Geometry check sheet. Reference: the model listing, model coordinates, mm. Face numbers are marked on the shaded views. A direction names the side the tool comes from. Give positions to 0.01 mm unless a question says otherwise; leave off trailing zeros. Write each loop counter-clockwise with the first axis right and the second up, starting at its lowest first coordinate (ties: lowest second). Pieces come first, ordered by that corner, then holes. Notation, with made-up numbers: (36.25, 36.5) -> (95.25, 36.5) arc R29 ccw to (95.25, 61.5) -> close; hole circle Ø5 at (-35.5, 89). An arc over 180 degrees is marked (long way). One line per item, written item: value.
from build123d import *

# Parameters (mm, degrees)
F0_W      = 200
F0_H      = 56.94
F0_W_2    = 5
F0_H_2    = 4.2824763805
F1_DEPTH  = 0.5
F2_DEPTH  = 0.501
F3_W      = 1
F3_H      = 24.6360383326
F4_DEPTH  = 6
F6_DEPTH  = 150.001
F8_W      = 1
F8_H      = 56.94
F9_DEPTH  = 20
F7_W      = 1
F7_H      = 56.94
F10_DEPTH = 20
F11_W     = 198
F11_H     = 1
F12_DEPTH = 20
F13_W     = 198
F13_H     = 1
F14_DEPTH = 20


with BuildPart() as f1:
    # F0 (on Top) → F1 (new body, symmetric)
    with BuildSketch(Plane.XY):
        Rectangle(F0_W, F0_H)
        with Locations((-60, 11.3287618098)):
            Rectangle(F0_W_2, F0_H_2, mode=Mode.SUBTRACT)
        with Locations((-40, 11.3287618098)):
            Rectangle(F0_W_2, F0_H_2, mode=Mode.SUBTRACT)
        with Locations((-20, 11.3287618098)):
            Rectangle(F0_W_2, F0_H_2, mode=Mode.SUBTRACT)
        with Locations((0, 11.3287618098)):
            Rectangle(F0_W_2, F0_H_2, mode=Mode.SUBTRACT)
        with Locations((20, 11.3287618098)):
            Rectangle(F0_W_2, F0_H_2, mode=Mode.SUBTRACT)
        with Locations((40, 11.3287618098)):
            Rectangle(F0_W_2, F0_H_2, mode=Mode.SUBTRACT)
        with Locations((60, 11.3287618098)):
            Rectangle(F0_W_2, F0_H_2, mode=Mode.SUBTRACT)
    extrude(amount=F1_DEPTH, both=True)

    # F0 (on Top) → F2 (cut, through all)
    with BuildSketch(Plane.XY):
        Rectangle(F0_W, F0_H)
        with Locations((-60, 11.3287618098)):
            Rectangle(F0_W_2, F0_H_2, mode=Mode.SUBTRACT)
        with Locations((-40, 11.3287618098)):
            Rectangle(F0_W_2, F0_H_2, mode=Mode.SUBTRACT)
        with Locations((-20, 11.3287618098)):
            Rectangle(F0_W_2, F0_H_2, mode=Mode.SUBTRACT)
        with Locations((0, 11.3287618098)):
            Rectangle(F0_W_2, F0_H_2, mode=Mode.SUBTRACT)
        with Locations((20, 11.3287618098)):
            Rectangle(F0_W_2, F0_H_2, mode=Mode.SUBTRACT)
        with Locations((40, 11.3287618098)):
            Rectangle(F0_W_2, F0_H_2, mode=Mode.SUBTRACT)
        with Locations((60, 11.3287618098)):
            Rectangle(F0_W_2, F0_H_2, mode=Mode.SUBTRACT)
    extrude(amount=-F2_DEPTH, mode=Mode.SUBTRACT)

    # F3 (on face) → F4 (join)
    with BuildSketch(Plane(origin=(0, 0, 0), x_dir=(1, 0, 0), z_dir=(0, 0, -1))):
        with Locations((-49.5, 10.1304955468)):
            Rectangle(F3_W, F3_H)
        with Locations((65.5, 10.1304955468)):
            Rectangle(F3_W, F3_H)
    extrude(amount=F4_DEPTH)

    # F5 (on face) → F6 (cut, through all)
    with BuildSketch(Plane(origin=(-50, 0, 0), x_dir=(0, -1, 0), z_dir=(-1, 0, 0))):
        with BuildLine():
            Line((-2.1875236195, -6), (22.448514713, -6))
            add(Edge.make_bspline(
                [(22.448514713, -6), (18.0848203599, -3.1530638225), (10.0274980374, -1.3176856102), (2.3821657524, -3.011564957), (-2.1875236195, -6)],
                knots=[0, 0, 0, 0, 0.5, 1, 1, 1, 1], degree=3))
        make_face()
    extrude(amount=-F6_DEPTH, mode=Mode.SUBTRACT)

    # F8 (on face) → F9 (join)
    with BuildSketch(Plane(origin=(0, 0, 0), x_dir=(1, 0, 0), z_dir=(0, 0, -1))):
        with Locations((99.5, 0)):
            Rectangle(F8_W, F8_H)
    extrude(amount=F9_DEPTH)

    # F7 (on face) → F10 (join)
    with BuildSketch(Plane(origin=(0, 0, 0), x_dir=(1, 0, 0), z_dir=(0, 0, -1))):
        with Locations((-99.5, 0)):
            Rectangle(F7_W, F7_H)
    extrude(amount=F10_DEPTH)

    # F11 (on face) → F12 (join)
    with BuildSketch(Plane(origin=(0, 0, 0), x_dir=(1, 0, 0), z_dir=(0, 0, -1))):
        with Locations((0, 27.97)):
            Rectangle(F11_W, F11_H)
    extrude(amount=F12_DEPTH)

    # F13 (on face) → F14 (join)
    with BuildSketch(Plane(origin=(0, 0, 0), x_dir=(1, 0, 0), z_dir=(0, 0, -1))):
        with Locations((0, -27.97)):
            Rectangle(F13_W, F13_H)
    extrude(amount=F14_DEPTH)


solid = f1.part
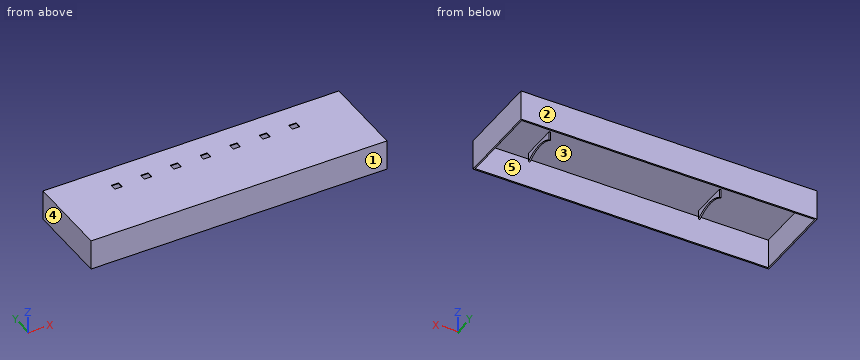
1) Tool access check on the marked faces 4 and 5. Record the directions out of +Z, -Z, +X, -X, +Y, -Y that give a thin tool (end or side, any length) a straight path to the whole face; none if there is none.
Verdict:
face 4: +Z, -Z, -X, +Y, -Y
face 5: -Z
2) Sectioned sample at C-C on y = 18. Record the cut outline in (x, z), plus the area to 3 significant figures.
Verdict:
outline: (-100, -20) -> (-99, -20) -> (-99, 0) -> (99, 0) -> (99, -20) -> (100, -20) -> (100, 0.5) -> (-100, 0.5) -> close
area: 140 mm^2
3) Sectioned sample at A-A on z = -14.5. Record the cut outline in (x, y).
Verdict:
outline: (-100, -28.47) -> (100, -28.47) -> (100, 28.47) -> (-100, 28.47) -> close; hole (-99, -27.47) -> (99, -27.47) -> (99, 27.47) -> (-99, 27.47) -> close
4) Scan lines: probe 1 along X at (y, z) = (-22, -5.25); probe 2 along Y at (x, z) = (-71.5, -11); probe 3 along X at (y, z) = (18, -6.25). Record each from-to range of solid material in increasing order.
Verdict:
probe 1: -100 to -99, -50 to -49, 65 to 66, 99 to 100
probe 2: -28.47 to -27.47, 27.47 to 28.47
probe 3: -100 to -99, 99 to 100
5) Sectioned sample at B-B on x = -55.5. Record the cut outline in (y, z).
Verdict:
outline: (-28.47, -20) -> (-27.47, -20) -> (-27.47, 0) -> (27.47, 0) -> (27.47, -20) -> (28.47, -20) -> (28.47, 0.5) -> (-28.47, 0.5) -> close
6) Mould release check, pull along Y, two halves, no side actions. Record for the marked faces 1, 2 and 3: released by +Y, released by -Y, zero draft, split by the parting line, or undercut.
Verdict:
face 1: released by -Y
face 2: released by +Y
face 3: undercut
7) Depth check by flat-ended pin: pin 1 Ø3 at (x, y) = (-32.5, 6) entering from -Z. Enter the tip coordinate at first touch or a pass-through.
Verdict:
pin 1: z = 0
